Design review of the part shown in the three views and the two pictorial views. Dimensions are in mm from the part's minimum x, y and z. A direction names the side the tool comes from. Give positions to 0.01 mm unless a question says otherwise; leave off trailing zeros. Loops run counter-clockwise (first coordinate to the right, second up) from the corner with the lowest first, then second, coordinate; pieces in that order, holes last. Notation, with made-up numbers: (61, -36.75) - (96, -36.75) arc R26 cw to (96, -4.75) - close; hole circle Ø2 at (18.5, 13.25). An arc over 180 degrees is marked (long way). Put each result on its own line as item: value. Start each with the question number.
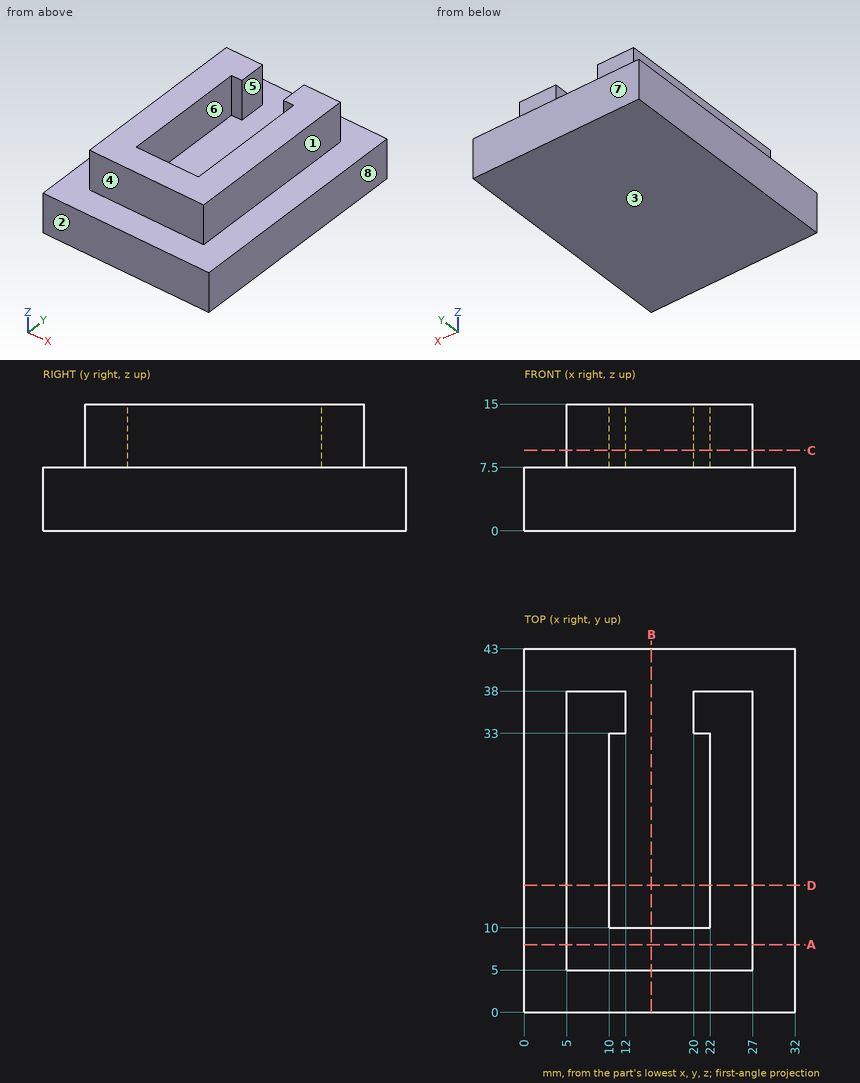
1) Insertion check: P1, Ø1, axis at x = 21, z = 11.5, coming from the -Y side; P2, Ø2, axis at x = 22, z = 9.5, coming from the +Y side; P3, Ø8, axis at y = 13.5, z = 12, coming from the +X side. Each pin has a flat end and moves straight along its axis. Give the tip position at first contact, or say it passes through.
2) Wall thickness on probe 1 along X at (y, z) = (20.5, 8); probe 2 along X at (y, z) = (36, 13.25); probe 3 along Z at (x, y) = (10, 41): over which ranges is each line inside the solid? List them lowest first.
3) Take a section at A-A on y = 8. State the section outline as (x, z) points.
4) Mouldability with a two-part tool opening along Y and no side actions: class the marked faces 6, 7 and 8 as released by +Y, released by -Y, zero draft, split by the parting line, or undercut.
5) Machinability: for the marked faces 1, 2, 3, 4 and 5, which of the approach directions +Z, -Z, +X, -X, +Y, -Y give a long, thin tool a straight path to every point of the face, cutting with its end or side? Answer none if there is none.
6) Take a section at D-D on y = 15. State the section outline as (x, z) points, and give its area (3 significant figures).
7) Take a section at C-C on z = 9.5. State the section outline as (x, y) points, and give its area (3 significant figures).
8) Take a section at B-B on x = 15. State the section outline as (y, z) points.
Answers follow:
1. P1: y = 5
1. P2: y = 38
1. P3: x = 27
2. probe 1: 5 to 10, 22 to 27
2. probe 2: 5 to 12, 20 to 27
2. probe 3: 0 to 7.5
3. outline: (0, 0) - (32, 0) - (32, 7.5) - (27, 7.5) - (27, 15) - (5, 15) - (5, 7.5) - (0, 7.5) - close
4. face 6: undercut
4. face 7: released by +Y
4. face 8: zero draft
5. face 1: +Z, +X, +Y, -Y
5. face 2: +Z, -Z, +X, -X, -Y
5. face 3: -Z, +X, -X, +Y, -Y
5. face 4: +Z, +X, -X, -Y
5. face 5: +Z, +Y
6. outline: (0, 0) - (32, 0) - (32, 7.5) - (27, 7.5) - (27, 15) - (22, 15) - (22, 7.5) - (10, 7.5) - (10, 15) - (5, 15) - (5, 7.5) - (0, 7.5) - close
6. area: 315 mm2
7. outline: (5, 5) - (27, 5) - (27, 38) - (20, 38) - (20, 33) - (22, 33) - (22, 10) - (10, 10) - (10, 33) - (12, 33) - (12, 38) - (5, 38) - close
7. area: 410 mm2
8. outline: (0, 0) - (43, 0) - (43, 7.5) - (10, 7.5) - (10, 15) - (5, 15) - (5, 7.5) - (0, 7.5) - close
